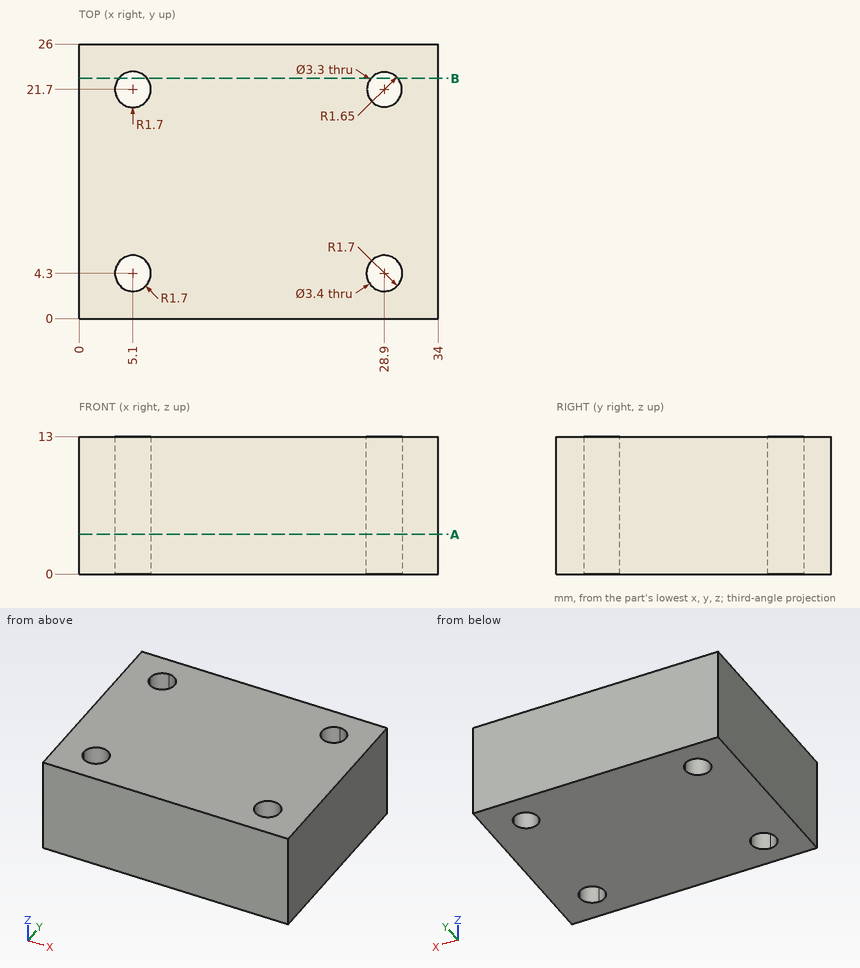
Can you work these out from the drawing? Everything is in mm from the part's minimum corner. Round coordinates to 2 decimals unless told otherwise and drop trailing zeros. Order: outer loops, then holes, each group sorted by start corner. A loop starts at its lowest first (then second) coordinate and runs counter-clockwise, first axis right, second up. Notation, with made-up numbers: M 87,27 L 118,27 A24 ccw 118,47 Z; hole C 27,88.5 d3. An arc over 180 degrees is marked long. Answer as CSV lines item,"result".
Item 1: Please list where these lines run through material, in increasing order: L1, parallel to X at y = 21.7, z = 10.5; L2, parallel to Y at x = 28.9, z = 3.5; L3, parallel to X at y = 4, z = 1.25. Write a range as [from, to].
From the geometry:
L1,"[0, 3.4], [6.8, 27.25], [30.55, 34]"
L2,"[0, 2.6], [6, 20.05], [23.35, 26]"
L3,"[0, 3.43], [6.77, 27.23], [30.57, 34]"
Item 2: Imagine slicing it at B-B on y = 22.75. List the corners of the cut face in (x, z) for me.
From the geometry:
outline,"M 0,0 L 3.76,0 L 3.76,13 L 0,13 Z; M 6.44,0 L 27.63,0 L 27.63,13 L 6.44,13 Z; M 30.17,0 L 34,0 L 34,13 L 30.17,13 Z"
Item 3: Imagine slicing it at A-A on z = 3.75. List the corners of the cut face in (x, y) for me, and give its area (3 significant figures).
From the geometry:
outline,"M 0,0 L 34,0 L 34,26 L 0,26 Z; hole M 3.4,4.3 A1.7 ccw 5.1,2.6 A1.7 ccw 6.8,4.3 A1.7 ccw Z; hole M 3.4,21.7 A1.7 ccw 6.8,21.7 A1.7 ccw 5.1,23.4 A1.7 ccw Z; hole C 28.9,21.7 d3.3; hole M 28.9,2.6 A1.7 ccw 30.6,4.3 A1.7 ccw long Z"
area,"848 mm2"
